The drawing under review shows one solid part. Ordinate dimensions are in mm from its lowest x, y, z. Give positions to 0.01 mm unless a question says otherwise; leave off trailing zeros. Loops run counter-clockwise (first coordinate to the right, second up) from the corner with the lowest first, then second, coordinate; pieces in that order, holes last. Notation, with made-up numbers: M -16,-16.5 L -5,-16.5 A20 ccw -5,8.5 Z; hole C -7,20.5 d11. An arc over 180 degrees is marked long. Put each result on its own line as item: value. Start each with the question number.
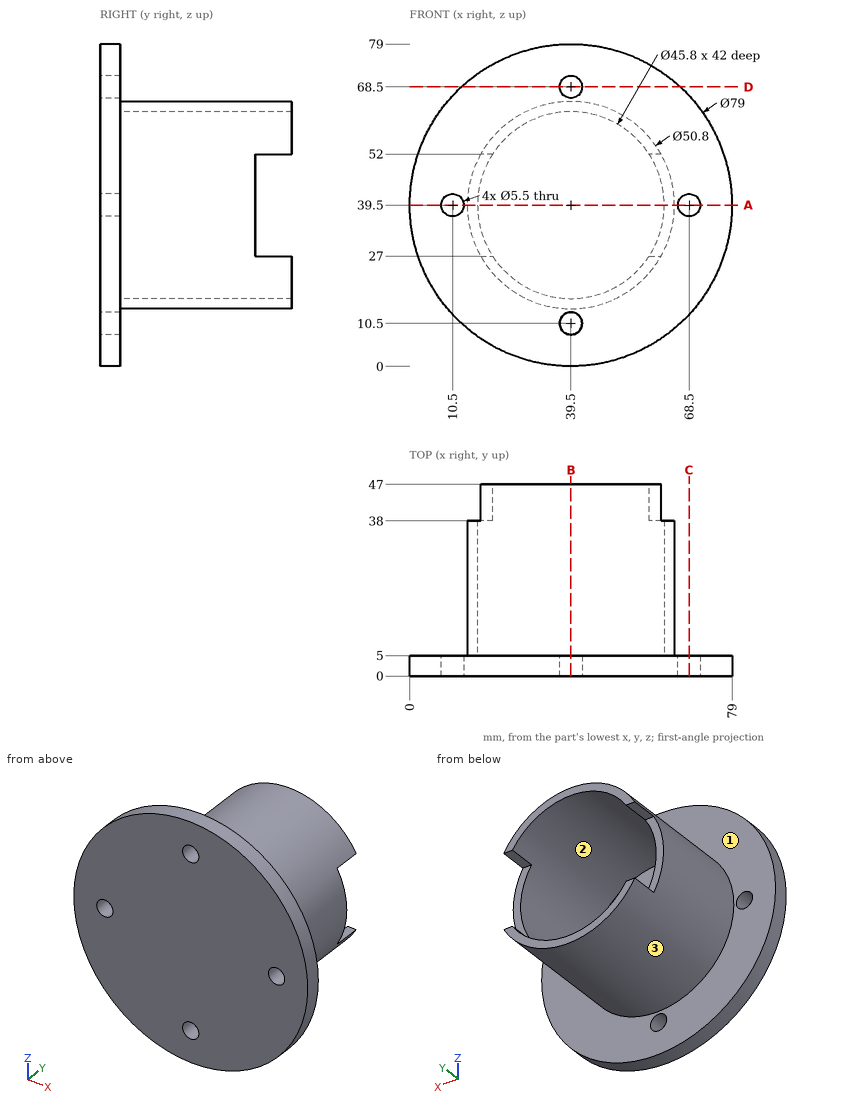
Item 1: Clearance check with flat-ended pins moving along their axes: pin 1 Ø4.5 at (x, z) = (39.5, 10.5) entering from -Y; pin 2 Ø6 at (y, z) = (22.5, 16) entering from +X; pin 3 Ø1 at (x, y) = (35.5, 14.5) entering from +Z; pin 4 Ø8 at (x, z) = (51, 41.5) entering from -Y. State where each tip first meets the part, or that it passes through.
Item 2: Consider section D-D, the plane z = 68.5. Write out the cut boundary in (x, y), plus the area to 3 significant figures.
Item 3: To check wall thickness, follow L1, parallel to Z at x = 39.5, y = 27; L2, parallel to Y at x = 16.5, z = 63. State the ranges of each line that lie inside material, in increasing order. Write a range as [from, to].
Item 4: Consider section A-A, the plane z = 39.5. Write out the cut boundary in (x, y), plus the area to 3 significant figures.
Item 5: Draft analysis for pull direction X (two halves, no side actions). For the marked faces 1, 2 and 3, state which applies: +X half, -X half, draft (parallel to the pull), parting line (faces both ways), or undercut.
Item 6: Consider section C-C, the plane x = 68.5. Write out the cut boundary in (y, z), plus the area to 3 significant figures.
Item 7: Consider section B-B, the plane x = 39.5. Write out the cut boundary in (y, z), plus the area to 3 significant figures.
Report:
1. pin 1: through
1. pin 2: x = 54.5
1. pin 3: z = 64.66
1. pin 4: y = 0
2. outline: M 12.68,0 L 36.75,0 L 36.75,5 L 12.68,5 Z; M 42.25,0 L 66.32,0 L 66.32,5 L 42.25,5 Z
2. area: 241 mm²
3. L1: [14.1, 16.6], [62.4, 64.9]
3. L2: [0, 5]
4. outline: M 0,0 L 7.75,0 L 7.75,5 L 0,5 Z; M 13.25,0 L 65.75,0 L 65.75,5 L 64.9,5 L 64.9,38 L 62.4,38 L 62.4,5 L 16.6,5 L 16.6,38 L 14.1,38 L 14.1,5 L 13.25,5 Z; M 71.25,0 L 79,0 L 79,5 L 71.25,5 Z
4. area: 505 mm²
5. face 1: draft
5. face 2: undercut
5. face 3: parting line
6. outline: M 0,12.68 L 5,12.68 L 5,36.75 L 0,36.75 Z; M 0,42.25 L 5,42.25 L 5,66.32 L 0,66.32 Z
6. area: 241 mm²
7. outline: M 0,0 L 5,0 L 5,7.75 L 0,7.75 Z; M 0,13.25 L 5,13.25 L 5,14.1 L 47,14.1 L 47,16.6 L 5,16.6 L 5,62.4 L 47,62.4 L 47,64.9 L 5,64.9 L 5,65.75 L 0,65.75 Z; M 0,71.25 L 5,71.25 L 5,79 L 0,79 Z
7. area: 550 mm²
